Answer from the drawing. Dimensions are ordinates in mm from the lowest x, y and z of the part. A direction names the side the tool comes from. Coordinates: 2 decimals unless noted, no trailing zeros. Write each loop counter-clockwise with the first axis right and the second up, starting at its lowest first coordinate (ties: lowest second). Pieces come first, ordered by that corner, then holes.
(1) The part is cut by section A-A on z = 37.5. Determine the outline of the cut face in (x, y).
(2) The part is cut by section C-C on y = 20. Determine the outline of the cut face in (x, z), plus the area to 3 significant figures.
(3) Straight lines are drawn through the part: line 1 (X direction, y = 28, z = 37) (1 decimal); line 2 (Z direction, x = 37.5, y = 10); line 3 (Z direction, x = 105, y = 21.5). For each, find the intervals that lie inside material, in ascending order.
(4) For a pull along Z with two mould halves and no side action, classify the marked faces 1, 2 and 3 as +Z half, -Z half, draft (parallel to the pull), parting line (faces both ways), or undercut.
(5) Which of the six approach directions +Z, -Z, +X, -X, +Y, -Y give full straight-line access (tool end or side, diameter ignored) to the marked faces 4 and 5?
(6) The part is cut by section D-D on x = 89. Determine the outline of the cut face in (y, z).
(7) The part is cut by section B-B on x = 37.5. Determine the outline of the cut face in (y, z), plus the area to 4 significant figures.
(8) Given P1, Ø1, axis at x = 80.5, y = 10, coming from the +Z side; P2, Ø1, axis at y = 23.5, z = 31, coming from the -X side; P3, Ø12, axis at x = 40, y = 11.5, coming from the +Z side; P4, Ø8, axis at x = 55.5, z = 46.5, coming from the -Y side, each flat-ended and moving along its own axis, determine where each tip first touches the part or whether it passes through.
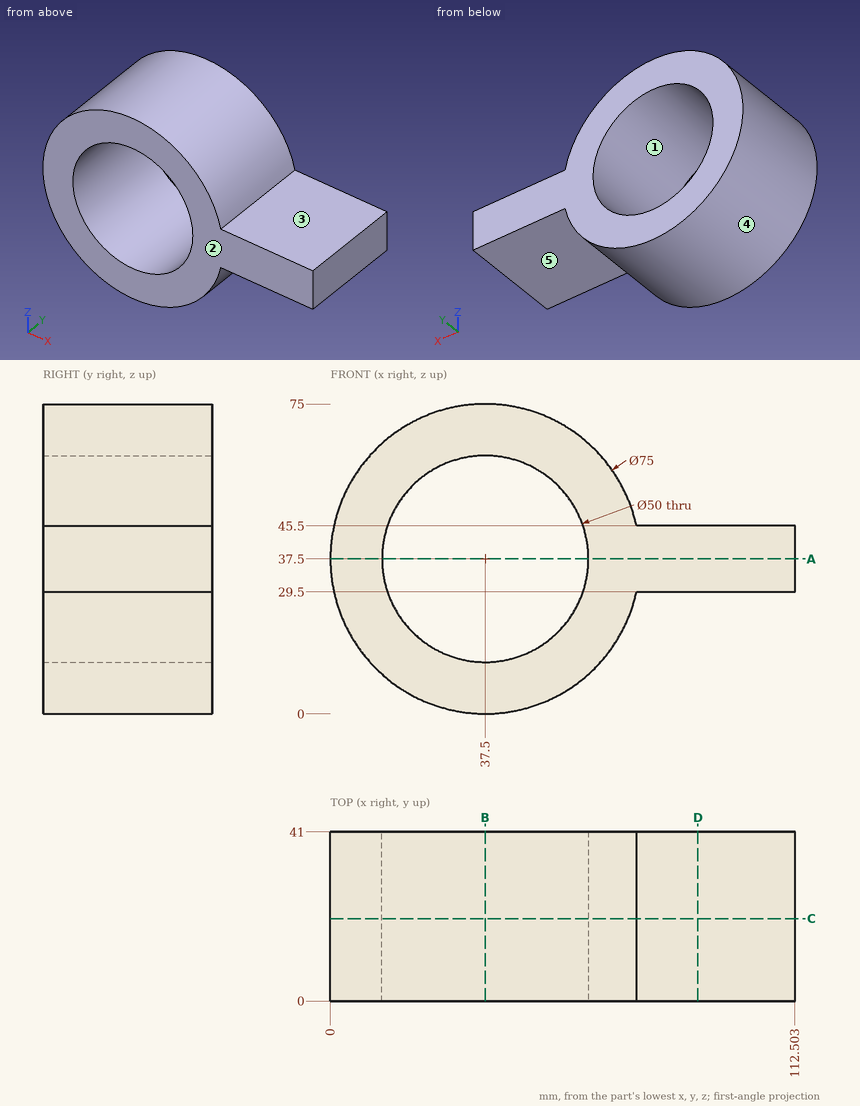
Model answer:
1. outline: (0, 0) - (12.5, 0) - (12.5, 41) - (0, 41) - close; (62.5, 0) - (112.5, 0) - (112.5, 41) - (62.5, 41) - close
2. outline: (74.14, 29.5) - (112.5, 29.5) - (112.5, 45.5) - (74.14, 45.5) arc R37.5 ccw (long way) to start; hole circle Ø50 at (37.5, 37.5)
2. area: 3,060 mm2
3. line 1: x = 0 to 12.5, 62.5 to 112.5
3. line 2: z = 0 to 12.5, 62.5 to 75
3. line 3: z = 29.5 to 45.5
4. face 1: undercut
4. face 2: draft
4. face 3: +Z half
5. face 4: +Y, -Y
5. face 5: -Z, +X, +Y, -Y
6. outline: (0, 29.5) - (41, 29.5) - (41, 45.5) - (0, 45.5) - close
7. outline: (0, 0) - (41, 0) - (41, 12.5) - (0, 12.5) - close; (0, 62.5) - (41, 62.5) - (41, 75) - (0, 75) - close
7. area: 1,025 mm2
8. P1: stops at z = 45.5
8. P2: stops at x = 0.48
8. P3: stops at z = 75
8. P4: passes through
